Source: CAD feature listing. Evaluate the final solid. Frame: model axes, mm. Face numbers are marked on the shaded views. A direction names the side the tool comes from. Round coordinates to 2 decimals unless told otherwise and drop trailing zeros. Loops run counter-clockwise (first coordinate to the right, second up) from the corner with the lowest first, then second, coordinate; pieces in that order, holes last. Notation, with made-up numbers: (14.5, 86.5) - (28.5, 86.5) arc R15 cw to (28.5, 98.5) - close; hole circle Ø9 at (25, -10.5). An arc over 180 degrees is marked (long way). One line per question, with ' | ' between items. Start each with the question number.
1. Cut plane C-C (x = 0.75). Return loops of the section in (y, z).
2. Cut plane A-A (z = -8). Return loops of the section in (x, y).
3. Ray query, line 1 (Y direction, x = -3, z = 0.5); line 2 (Y direction, x = -4.25, z = 1.75); line 3 (X direction, y = 3, z = -3.5). Return the intervals inside material, ascending.
4. Cut plane B-B (x = -1.5). Return loops of the section in (y, z), then the cut area to 3 significant figures.
5. Mould query, pull axis X, two halves, no side actions, for the marked faces 1, 2, 3 and 4. Classes: pulls with the +X half, pulls with the -X half, needs draft (parallel to the pull), parting line crosses it, or undercut.
6. Cut plane D-D (z = -3.25). Return loops of the section in (x, y).
7. Pin query (flat end, axial travel): pin 1 (3 mm diameter, centred on x = -2.42, z = -3.68, fed in from +Y); pin 2 (1 mm diameter, centred on x = -3, y = 8, fed in from -Z); pin 3 (2 mm diameter, centred on y = 12.5, z = -7.5, fed in from +X). Return the tip coordinate at first contact, or that it passes through.
8. Access query for the marked faces 5, 6 and 7. Directions: +Z, -Z, +X, -X, +Y, -Y. A direction counts if a zero-diameter tool reaches every point of the face in a straight line with its end or side. Return the directions, or none.
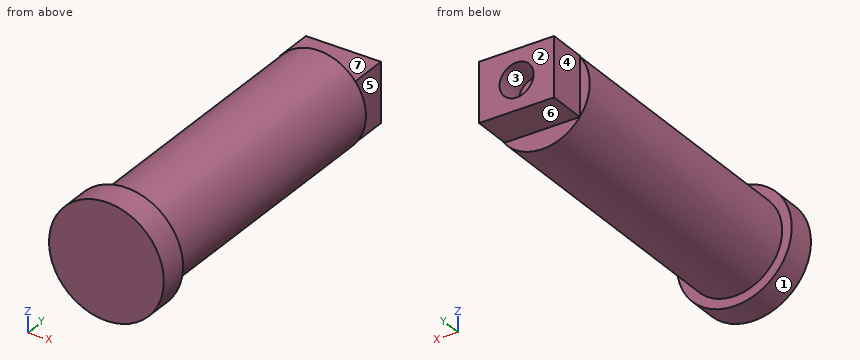
```python
from build123d import *

# Parameters (mm, degrees)
SKETCH1_R           = 5
BOSS_EXTRUDE2_DEPTH = 30
SKETCH2_W           = 7.845289229
SKETCH2_H           = 6.199593877
BOSS_EXTRUDE3_DEPTH = 4
SKETCH3_R           = 1.774695969
CUT_EXTRUDE1_DEPTH  = 3
SKETCH4_R           = 6
BOSS_EXTRUDE4_DEPTH = 3


with BuildPart() as part:
    # Sketch1 → Boss-Extrude2 (new body)
    with BuildSketch(Plane(origin=(0, 0, 0), x_dir=(1, 0, 0), z_dir=(0, 1, 0))):
        with Locations(Location((-2.376457655, 3.696711907, 0), (0, 0, 270))):
            Circle(SKETCH1_R)
    extrude(amount=BOSS_EXTRUDE2_DEPTH)

    # Sketch2 → Boss-Extrude3 (add)
    with BuildSketch(Plane(origin=(0, 30, 0), x_dir=(1, 0, 0), z_dir=(0, 1, 0))):
        with Locations((-2.416245544, 3.646362238)):
            Rectangle(SKETCH2_W, SKETCH2_H)
    extrude(amount=BOSS_EXTRUDE3_DEPTH)

    # Sketch3 → Cut-Extrude1 (cut)
    with BuildSketch(Plane(origin=(0, 34, 0), x_dir=(1, 0, 0), z_dir=(0, 1, 0))):
        with Locations(Location((-2.415547682, 3.681180673, 0), (0, 0, 270))):
            Circle(SKETCH3_R)
    extrude(amount=-CUT_EXTRUDE1_DEPTH, mode=Mode.SUBTRACT)

    # Sketch4 → Boss-Extrude4 (add)
    with BuildSketch(Plane(origin=(0, 0, 0), x_dir=(-1, 0, 0), z_dir=(0, -1, 0))):
        with Locations(Location((2.376457655, 3.696711907, 0), (0, 0, 90))):
            Circle(SKETCH4_R)
    extrude(amount=BOSS_EXTRUDE4_DEPTH)


solid = part.part
```
Answers follow:
1) outline: (-3, -8.82) - (0, -8.82) - (0, -7.6) - (30, -7.6) - (30, -6.75) - (34, -6.75) - (34, -0.55) - (30, -0.55) - (30, 0.21) - (0, 0.21) - (0, 1.42) - (-3, 1.42) - close
2) outline: (-6.56, -3) - (1.8, -3) - (1.8, 0) - (0.17, 0) - (0.17, 30) - (-4.92, 30) - (-4.92, 0) - (-6.56, 0) - close
3) line 1: y = -3 to 30 | line 2: y = -3 to 0 | line 3: x = -7.37 to 2.62
4) outline: (-3, -9.63) - (0, -9.63) - (0, -8.62) - (30, -8.62) - (30, -6.75) - (34, -6.75) - (34, -5.2) - (31, -5.2) - (31, -2.16) - (34, -2.16) - (34, -0.55) - (30, -0.55) - (30, 1.23) - (0, 1.23) - (0, 2.24) - (-3, 2.24) - close | area: 347 mm2
5) face 1: parting line crosses it | face 2: needs draft | face 3: undercut | face 4: pulls with the -X half
6) outline: (-8.36, -3) - (3.61, -3) - (3.61, 0) - (2.6, 0) - (2.6, 30) - (1.51, 30) - (1.51, 34) - (-0.69, 34) - (-0.69, 31) - (-4.14, 31) - (-4.14, 34) - (-6.34, 34) - (-6.34, 30) - (-7.36, 30) - (-7.36, 0) - (-8.36, 0) - close
7) pin 1: stops at y = 31 | pin 2: stops at z = -8.7 | pin 3: stops at x = 1.76
8) face 5: +Z, -Z, +X, +Y | face 6: -Z, +X, -X, +Y | face 7: +Z, +X, -X, +Y
